```python
from build123d import *

# Parameters (mm, degrees)
SKETCH1_R           = 10
SKETCH1_R_2         = 20
SKETCH1_R_3         = 2
SKETCH1_R_4         = 1.5
BOSS_EXTRUDE1_DEPTH = 4
CUT_EXTRUDE1_DEPTH  = 10


with BuildPart() as part:
    # Sketch1 → Boss-Extrude1 (new body)
    with BuildSketch(Plane(origin=(0, 0, 0), x_dir=(0, 0, -1), z_dir=(1, 0, 0))):
        with BuildLine():
            Line((8.06779661, 33.028936675), (63.745762712, 19.428786279))
            ThreePointArc((63.745762712, 19.428786279), (79, 0), (63.745762712, -19.428786279))
            Line((63.745762712, -19.428786279), (8.06779661, -33.028936675))
            ThreePointArc((8.06779661, -33.028936675), (-34, 0), (8.06779661, 33.028936675))
        make_face()
        with Locations((59, 0)):
            Circle(SKETCH1_R, mode=Mode.SUBTRACT)
        Circle(SKETCH1_R_2, mode=Mode.SUBTRACT)
        with Locations((0, 29)):
            Circle(SKETCH1_R_3, mode=Mode.SUBTRACT)
        with Locations((20.506096654, 20.506096654)):
            Circle(SKETCH1_R_3, mode=Mode.SUBTRACT)
        with Locations((29, 0)):
            Circle(SKETCH1_R_3, mode=Mode.SUBTRACT)
        with Locations((20.506096654, -20.506096654)):
            Circle(SKETCH1_R_3, mode=Mode.SUBTRACT)
        with Locations((0, -29)):
            Circle(SKETCH1_R_3, mode=Mode.SUBTRACT)
        with Locations((-20.506096654, -20.506096654)):
            Circle(SKETCH1_R_3, mode=Mode.SUBTRACT)
        with Locations((-29, 0)):
            Circle(SKETCH1_R_3, mode=Mode.SUBTRACT)
        with Locations((-20.506096654, 20.506096654)):
            Circle(SKETCH1_R_3, mode=Mode.SUBTRACT)
        with Locations((49.807611845, 9.192388155)):
            Circle(SKETCH1_R_4, mode=Mode.SUBTRACT)
        with Locations((68.192388155, 9.192388155)):
            Circle(SKETCH1_R_4, mode=Mode.SUBTRACT)
        with Locations((68.192388155, -9.192388155)):
            Circle(SKETCH1_R_4, mode=Mode.SUBTRACT)
        with Locations((49.807611845, -9.192388155)):
            Circle(SKETCH1_R_4, mode=Mode.SUBTRACT)
    extrude(amount=BOSS_EXTRUDE1_DEPTH)

    # Sketch2 → Cut-Extrude1 (cut)
    with BuildSketch(Plane.ZY):
        with BuildLine():
            ThreePointArc((-28.995147078, -7.929410218), (-35.694510355, -8.730689231), (-39.865085734, -14.034444257))
            ThreePointArc((-39.865085734, -14.034444257), (-38.826287735, -15.884011427), (-36.976720565, -14.845213428))
            ThreePointArc((-36.976720565, -14.845213428), (-34.225428136, -11.346372207), (-29.805916249, -10.817775387))
            ThreePointArc((-29.805916249, -10.817775387), (-27.956349079, -9.778977388), (-28.995147078, -7.929410218))
        make_face()
    extrude(amount=-CUT_EXTRUDE1_DEPTH, mode=Mode.SUBTRACT)


solid = part.part
```
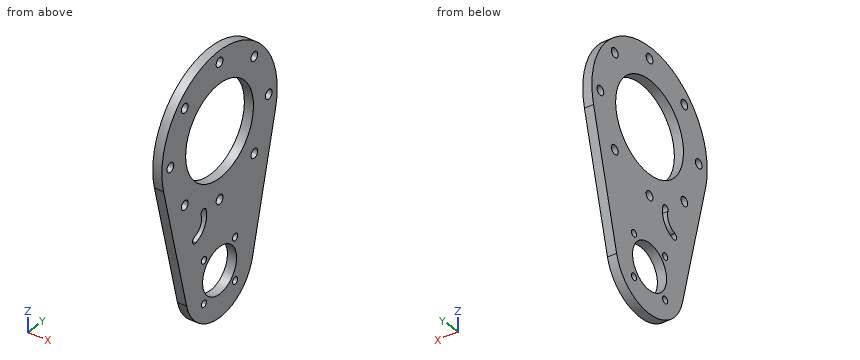
The model under review builds one solid part; all positions refer to its coordinate system, in mm. Give positions to 0.01 mm unless a question says otherwise; leave off trailing zeros. Write each loop counter-clockwise with the first axis right and the second up, starting at its lowest first coordinate (ties: lowest second). Pieces come first, ordered by that corner, then holes. Notation, with made-up numbers: (-28.5, 1.5) -> (-8.5, 1.5) arc R27 cw to (-8.5, 35.5) -> close; hole circle Ø2 at (75.25, -12). An arc over 180 degrees is marked (long way). Answer in a Markdown table with one row per item.
1) Add section C-C on z = -59. State the section outline as (x, y) points.
Worked answers:
| item | result |
|---|---|
| outline | (0, -20.59) -> (4, -20.59) -> (4, -10) -> (0, -10) -> close; (0, 10) -> (4, 10) -> (4, 20.59) -> (0, 20.59) -> close |
2) Add section B-B on z = 0. State the section outline as (x, y) points.
Worked answers:
| item | result |
|---|---|
| outline | (0, -34) -> (4, -34) -> (4, -31) -> (0, -31) -> close; (0, -27) -> (4, -27) -> (4, -20) -> (0, -20) -> close; (0, 20) -> (4, 20) -> (4, 27) -> (0, 27) -> close; (0, 31) -> (4, 31) -> (4, 34) -> (0, 34) -> close |
3) Add section A-A on y = 0. State the section outline as (x, z) points, plus the area to 3 significant figures.
Worked answers:
| item | result |
|---|---|
| outline | (0, -79) -> (4, -79) -> (4, -69) -> (0, -69) -> close; (0, -49) -> (4, -49) -> (4, -31) -> (0, -31) -> close; (0, -27) -> (4, -27) -> (4, -20) -> (0, -20) -> close; (0, 20) -> (4, 20) -> (4, 27) -> (0, 27) -> close; (0, 31) -> (4, 31) -> (4, 34) -> (0, 34) -> close |
| area | 180 mm² |
4) Add section D-D on y = 15. State the section outline as (x, z) points, plus the area to 3 significant figures.
Worked answers:
| item | result |
|---|---|
| outline | (0, -72.23) -> (4, -72.23) -> (4, -13.23) -> (0, -13.23) -> close; (0, 13.23) -> (4, 13.23) -> (4, 30.51) -> (0, 30.51) -> close |
| area | 305 mm² |
5) Clearance check with flat-ended pins moving along their axes: P1, Ø2, axis at x = 1.5, z = -58.5, coming from the -Y side; P2, Ø2, axis at x = 1, z = -55.5, coming from the -Y side; P3, Ø2, axis at x = 1.5, z = -6.5, coming from the -Y side. State where each tip first meets the part, or that it passes through.
Worked answers:
| item | result |
|---|---|
| P1 | y = -20.95 |
| P2 | y = -21.69 |
| P3 | y = -33.55 |
6) For L1, parallel to Z at x = 1.4, y = -3; L2, parallel to Z at x = 2.3, y = 9; L3, parallel to Z at x = 1.1, y = -1, list the stretches that pass through material, from the lowest coordinate up. Write a range as [from, to].
Worked answers:
| item | result |
|---|---|
| L1 | [-78.77, -68.54], [-49.46, -19.77], [19.77, 33.87] |
| L2 | [-76.86, -69.68], [-66.7, -63.36], [-54.64, -51.3], [-48.32, -17.86], [17.86, 32.79] |
| L3 | [-78.97, -68.95], [-49.05, -30.73], [-27.27, -19.97], [19.97, 27.27], [30.73, 33.99] |
